Geometry: final body of the model. Coordinates: model frame, mm. A direction names the side the tool comes from. Give positions to 0.01 mm unless a question says otherwise; leave off trailing zeros. Order: outer loops, then holes, each group sorted by start corner. A loop starts at its lowest first (then second) coordinate and runs counter-clockwise, first axis right, second up. Notation, with made-up numbers: (-8, 15) - (45, 15) arc R35 cw to (45, 52) - close; hole circle Ø3 at (1, 18). An arc over 180 degrees is marked (long way). Use one line per item in the form item = value.
from build123d import *

# Parameters (mm, degrees)
F0_R     = 11
F1_DEPTH = 3


with BuildPart() as f1:
    # F0 (on Top) → F1 (new body)
    with BuildSketch(Plane.XY):
        with BuildLine():
            ThreePointArc((15.224018, 8.630137), (15.18985, 8.690136), (15.155445, 8.75))
            ThreePointArc((15.155445, 8.75), (15.120804, 8.809728), (15.085927, 8.869318))
            ThreePointArc((15.085927, 8.869318), (11.574062, 19.543722), (12.801487, 30.71375))
            ThreePointArc((12.801487, 30.71375), (0, 48.5), (-12.801487, 30.71375))
            ThreePointArc((-12.801487, 30.71375), (-11.574062, 19.543722), (-15.085927, 8.869318))
            ThreePointArc((-15.085927, 8.869318), (-15.120804, 8.809728), (-15.155445, 8.75))
            ThreePointArc((-15.155445, 8.75), (-15.18985, 8.690136), (-15.224018, 8.630137))
            ThreePointArc((-15.224018, 8.630137), (-22.712391, 0.25157), (-32.999631, -4.270462))
            ThreePointArc((-32.999631, -4.270462), (-42.002232, -24.25), (-20.198144, -26.443288))
            ThreePointArc((-20.198144, -26.443288), (-11.138329, -19.795292), (-0.138091, -17.499455))
            ThreePointArc((-0.138091, -17.499455), (-0.069046, -17.499864), (0, -17.5))
            ThreePointArc((0, -17.5), (0.069046, -17.499864), (0.138091, -17.499455))
            ThreePointArc((0.138091, -17.499455), (11.138329, -19.795292), (20.198144, -26.443288))
            ThreePointArc((20.198144, -26.443288), (42.002232, -24.25), (32.999631, -4.270462))
            ThreePointArc((32.999631, -4.270462), (22.712391, 0.25157), (15.224018, 8.630137))
        make_face()
        with Locations((-30.310889, -17.5)):
            Circle(F0_R, mode=Mode.SUBTRACT)
        with Locations((30.310889, -17.5)):
            Circle(F0_R, mode=Mode.SUBTRACT)
        with BuildLine():
            ThreePointArc((-9.526279, 5.5), (0, 11), (9.526279, 5.5))
            ThreePointArc((9.526279, 5.5), (9.526279, -5.5), (0, -11))
            ThreePointArc((0, -11), (-9.526279, -5.5), (-9.526279, 5.5))
        make_face(mode=Mode.SUBTRACT)
        with Locations((0, 35)):
            Circle(F0_R, mode=Mode.SUBTRACT)
    extrude(amount=F1_DEPTH)


solid = f1.part
(1) Reachability of faces 4 (the face through (10.99, -19.73, 1.48)), 5 (the face through (-8.11, 42.43, 1.48)) from +Z, -Z, +X, -X, +Y, -Y: full face, straight path, thin tool, end or side. Return the list, or none.
Computed values:
face_4 = +Z, -Z, -Y
face_5 = +Z, -Z
(2) Cut plane C-C on z = 0.65. Output: boundary loops of the cut face in (x, y).
Computed values:
outline = (-33, -4.27) arc R13.5 ccw (long way) to (-20.2, -26.44) arc R26.5 cw to (-0.14, -17.5) arc R17.46 ccw to (0, -17.5) arc R17.46 ccw to (0.14, -17.5) arc R26.5 cw to (20.2, -26.44) arc R13.5 ccw (long way) to (33, -4.27) arc R26.5 cw to (15.22, 8.63) arc R17.48 ccw to (15.16, 8.75) arc R17.44 ccw to (15.09, 8.87) arc R26.5 cw to (12.8, 30.71) arc R13.5 ccw (long way) to (-12.8, 30.71) arc R26.5 cw to (-15.09, 8.87) arc R17.44 ccw to (-15.16, 8.75) arc R17.48 ccw to (-15.22, 8.63) arc R26.5 cw to start; hole circle Ø22 at (-30.31, -17.5); hole circle Ø22 at (0, 0); hole circle Ø22 at (0, 35); hole circle Ø22 at (30.31, -17.5)
(3) Cut plane B-B on x = -36.5. Output: boundary loops of the cut face in (y, z), plus the area to 3 significant figures.
Computed values:
outline = (-29.5, 0) - (-26.59, 0) - (-26.59, 3) - (-29.5, 3) - close; (-8.41, 0) - (-5.5, 0) - (-5.5, 3) - (-8.41, 3) - close
area = 17.4 mm²
(4) Cut plane A-A on y = -5.5. Output: boundary loops of the cut face in (x, z).
Computed values:
outline = (-36.5, 0) - (-9.53, 0) - (-9.53, 3) - (-36.5, 3) - close; (9.53, 0) - (36.5, 0) - (36.5, 3) - (9.53, 3) - close
(5) Cut plane D-D on y = 14.5. Output: boundary loops of the cut face in (x, z).
Computed values:
outline = (-12.6, 0) - (12.6, 0) - (12.6, 3) - (-12.6, 3) - close
(6) Contact query for a flat-ended pin moving along its axis: pin 1 Ø17.5 at (x, y) = (-30.31, -17.5) entering from +Z. Output: stop coordinate, or through.
Computed values:
pin_1 = through
(7) Ray query, line 1 along Y through (x, z) = (5, 1.35); line 2 along X through (y, z) = (-14.5, 1.1); line 3 along Y through (x, z) = (-8, 1.7). Return the intervals inside material, ascending.
Computed values:
line_1 = -17.91 to -9.8, 9.8 to 25.2, 44.8 to 47.54
line_2 = -43.47 to -40.89, -19.73 to 19.73, 40.89 to 43.47
line_3 = -18.63 to -7.55, 7.55 to 27.45, 42.55 to 45.87
(8) Pull-direction query (Y, two-part tool) for faces 1 (the face through (22.84, 0.16, 1.48)), 2 (the face through (-11.28, -19.86, 1.48)), 3 (the face through (-20.15, -21.71, 1.48)); classes: released by +Y, released by -Y, zero draft, split by the parting line, or undercut.
Computed values:
face_1 = released by +Y
face_2 = released by -Y
face_3 = undercut
